```python
from build123d import *

# Parameters (mm, degrees)
PAD010_DEPTH    = 20
SKETCH018_W     = 12.75
SKETCH018_H     = 10.8
POCKET006_DEPTH = 33.75
POCKET007_DEPTH = 50
SKETCH017_R     = 4.9
POCKET008_DEPTH = 30.001
SKETCH020_R     = 2.6
POCKET009_DEPTH = 20.001
SKETCH021_R     = 2.5
POCKET010_DEPTH = 31.086657
POCKET011_DEPTH = 10.8


with BuildPart() as part:
    # Sketch016 → Pad010 (new body, symmetric)
    with BuildSketch(Plane.YZ):
        Polygon((23.315383, 0), (0, 50), (-9.063078, 45.773817), (-20, 12), (-20, 0), align=None)
    extrude(amount=PAD010_DEPTH, both=True)

    # Sketch018 → Pocket006 (cut)
    with BuildSketch(Plane.XZ.offset(20)):
        with Locations((0, 5.4)):
            Rectangle(SKETCH018_W, SKETCH018_H)
    extrude(amount=-POCKET006_DEPTH, mode=Mode.SUBTRACT)

    # Sketch019 → Pocket007 (cut)
    with BuildSketch(Plane(origin=(0, 13, 5), x_dir=(1, 0, 0), z_dir=(0, -0.906308, -0.422618))):
        with BuildLine():
            Line((-29.407349, 60.205246), (-7, 60.205246))
            Line((-7, 60.205246), (-7, 24.801724))
            ThreePointArc((-19.801724, 12), (-10.749538, 15.749538), (-7, 24.801724))
            Line((-19.801724, 12), (-29.407349, 12))
            Line((-29.407349, 12), (-29.407349, 60.205246))
        make_face()
        with BuildLine():
            Line((7, 60.205246), (29.407349, 60.205246))
            Line((29.407349, 60.205246), (29.407349, 12))
            Line((29.407349, 12), (19.801724, 12))
            ThreePointArc((7, 24.801724), (10.749538, 15.749538), (19.801724, 12))
            Line((7, 24.801724), (7, 60.205246))
        make_face()
    extrude(amount=POCKET007_DEPTH, mode=Mode.SUBTRACT)

    # Sketch017 → Pocket008 (cut, through all)
    with BuildSketch(Plane.XY.offset(20)):
        with Locations((0, -6)):
            Circle(SKETCH017_R)
        with Locations((0, 8.5)):
            Circle(SKETCH017_R)
    extrude(amount=POCKET008_DEPTH, mode=Mode.SUBTRACT)

    # Sketch020 → Pocket009 (cut, through all)
    with BuildSketch(Plane.XY.offset(20)):
        with Locations((0, -6)):
            Circle(SKETCH020_R)
        with Locations((0, 8.5)):
            Circle(SKETCH020_R)
    extrude(amount=-POCKET009_DEPTH, mode=Mode.SUBTRACT)

    # Sketch021 → Pocket010 (cut, through all)
    with BuildSketch(Plane(origin=(0, 10, 5), x_dir=(1, 0, 0), z_dir=(0, -0.906308, -0.422618))):
        with Locations((15.5, 18.346014)):
            Circle(SKETCH021_R)
        with Locations((-15.5, 18.346014)):
            Circle(SKETCH021_R)
        with Locations((15.5, 40.846014)):
            Circle(SKETCH021_R)
        with Locations((-15.5, 40.846014)):
            Circle(SKETCH021_R)
    extrude(amount=-POCKET010_DEPTH, mode=Mode.SUBTRACT)

    # Sketch022 → Pocket011 (cut)
    with BuildSketch(Plane.XY):
        Polygon((-7.9, -20.114331), (7.9, -20.114331), (7.377167, -2.314331), (-7.377167, -2.314331), align=None)
    extrude(amount=POCKET011_DEPTH, mode=Mode.SUBTRACT)


with BuildPart() as part_1:
    # Body009 placement: moved
    add(part.part.moved(Location((30.5, -12, 2))))


solid = part_1.part
```
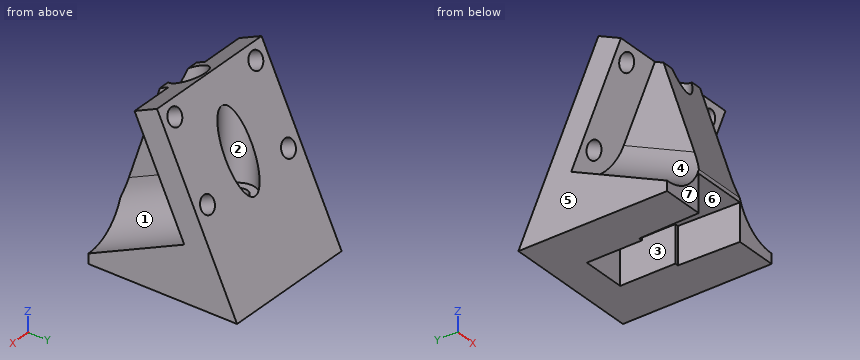
Model file for the job. Use its own axes, mm. Face numbers are marked on the shaded views. A direction names the side the tool comes from. Round coordinates to 2 decimals unless told otherwise and drop trailing zeros. Write each loop counter-clockwise with the first axis right and the second up, starting at its lowest first coordinate (ties: lowest second). Pieces come first, ordered by that corner, then holes. Notation, with made-up numbers: M -26,-25.75 L 11,-25.75 A27 cw 11,2.25 Z; hole C -26,15 d6. An arc over 180 degrees is marked long. Put each result on its own line as item: value.
Item 1: Mould opens along X. For the marked faces 5, 6 and 7 say: +X half, -X half, draft (parallel to the pull), parting line (faces both ways), or undercut.
Responses:
face 5: -X half
face 6: undercut
face 7: draft
Item 2: Cut at B-B (z = 42). List the corners of the cut face in (x, y).
Responses:
outline: M 10.5,-15.32 L 23.5,-15.32 L 23.5,-22.93 L 37.5,-22.93 L 37.5,-15.32 L 50.5,-15.32 L 50.5,-7.34 L 33.55,-7.34 A4.9 cw 27.45,-7.34 L 10.5,-7.34 Z; hole C 30.5,-18 d9.8
Item 3: Flat gauge pins, fed straight in: P1, Ø6, axis at x = 30.5, y = -18, coming from the -Z side; P2, Ø3, axis at x = 30.5, y = -2.5, coming from the +Z side; P3, Ø6, axis at x = 30.5, y = -3.5, coming from the +Z side; P4, Ø12, axis at x = 23, y = 6.5, coming from the +Z side. Where does each tip first touch, or does it go through?
Responses:
P1: z = 12.8
P2: through
P3: z = 22
P4: z = 25.19
Item 4: Cut at A-A (x = 47.5). List the corners of the cut face in (y, z), and give its area (3 significant figures).
Responses:
outline: M -32,2 L 11.32,2 L 0.11,26.02 L -6.44,22.96 L -4.2,18.16 L -32,5.19 Z; M -18.56,48.94 L -17.64,46.98 L -11.09,50.04 L -12,52 Z; M -15.95,43.36 L -8.13,26.59 L -1.58,29.65 L -9.39,46.41 Z
area: 659 mm²
Item 5: Probe L1, parallel to Z at x = 32, y = -1; L2, parallel to X at y = -14, z = 11 (3 decimals); L3, parallel to Y at x = 30, z = 17. List the from-to ranges inside material, lowest first. Write a range as from..to.
Responses:
L1: 12.8..22
L2: 10.5..24.125, 36.875..50.5
L3: -31.03..-20.55, -15.45..-6.05, -0.95..4.32
Item 6: Cut at D-D (z = 15). State how many separate pieces and enclosed holes the cut face has, and give its area (3 significant figures).
Responses:
separate pieces: 1
enclosed holes: 2
area: 1,040 mm²
Item 7: Cut at C-C (x = 29). List the corners of the cut face in (y, z).
Responses:
outline: M -32,12.8 L -20.12,12.8 L -20.12,22 L -22.66,22 L -22.66,42.83 L -32,14 Z; M -15.88,12.8 L -5.62,12.8 L -5.62,22 L -8.16,22 L -8.16,43.78 L -12,52 L -13.34,51.38 L -13.34,22 L -15.88,22 Z; M -1.38,12.8 L 1.75,12.8 L 1.75,2 L 11.32,2 L 1.16,23.77 L 1.16,22 L -1.38,22 Z
Item 8: Tool access for the marked faces 1, 2, 3 and 4: list every direction of +Z, -Z, +X, -X, +Y, -Y with a clear straight run to the whole face (end or side of a thin tool).
Responses:
face 1: +X, -Y
face 2: +Z
face 3: -Z, -Y
face 4: -X, -Y
